Input: dimensioned drawing with shaded views. Units: mm. Origin: part minimum x, y, z. Coordinates: 2 decimals unless noted, no trailing zeros. Order: outer loops, then holes, each group sorted by start corner. A loop starts at its lowest first (then second) coordinate and runs counter-clockwise, first axis right, second up. Notation, with made-up numbers: (88.5, 66) -> (95.5, 66) arc R25 cw to (95.5, 80) -> close; hole circle Ø11 at (70, -20). An arc over 180 degrees is marked (long way). Write item = value, one per line. Start each with the question number.
Item 1: Section query A-A (x = 38). Output: boundary loops of the cut face in (y, z), then the cut area to 3 significant figures.
Item 2: Section query D-D (x = 51). Output: boundary loops of the cut face in (y, z), then the cut area to 3 significant figures.
Item 3: Section query B-B (z = 38). Output: boundary loops of the cut face in (x, y).
Item 4: Contact query for flat-ended pins moving along their axis: pin 1 (5 mm diameter, centred on y = 7.5, z = 50, fed in from +X); pin 2 (3 mm diameter, centred on y = 5.5, z = 41.5, fed in from +X); pin 3 (1.5 mm diameter, centred on x = 61, y = 7, fed in from +Z) (1 decimal). Output: stop coordinate, or through.
Item 5: Section query C-C (z = 29). Output: boundary loops of the cut face in (x, y).
Item 6: Ray query, line 1 along X through (y, z) = (4.5, 38); line 2 along Z through (x, y) = (21.5, 8); line 3 along Z through (x, y) = (21, 1.75) (1 decimal). Return the intervals inside material, ascending. Write a range as [from, to].
Item 7: Mould query, pull axis Z, two halves, no side actions, for the marked faces 1, 2 and 3. Classes: released by +Z, released by -Z, zero draft, split by the parting line, or undercut.
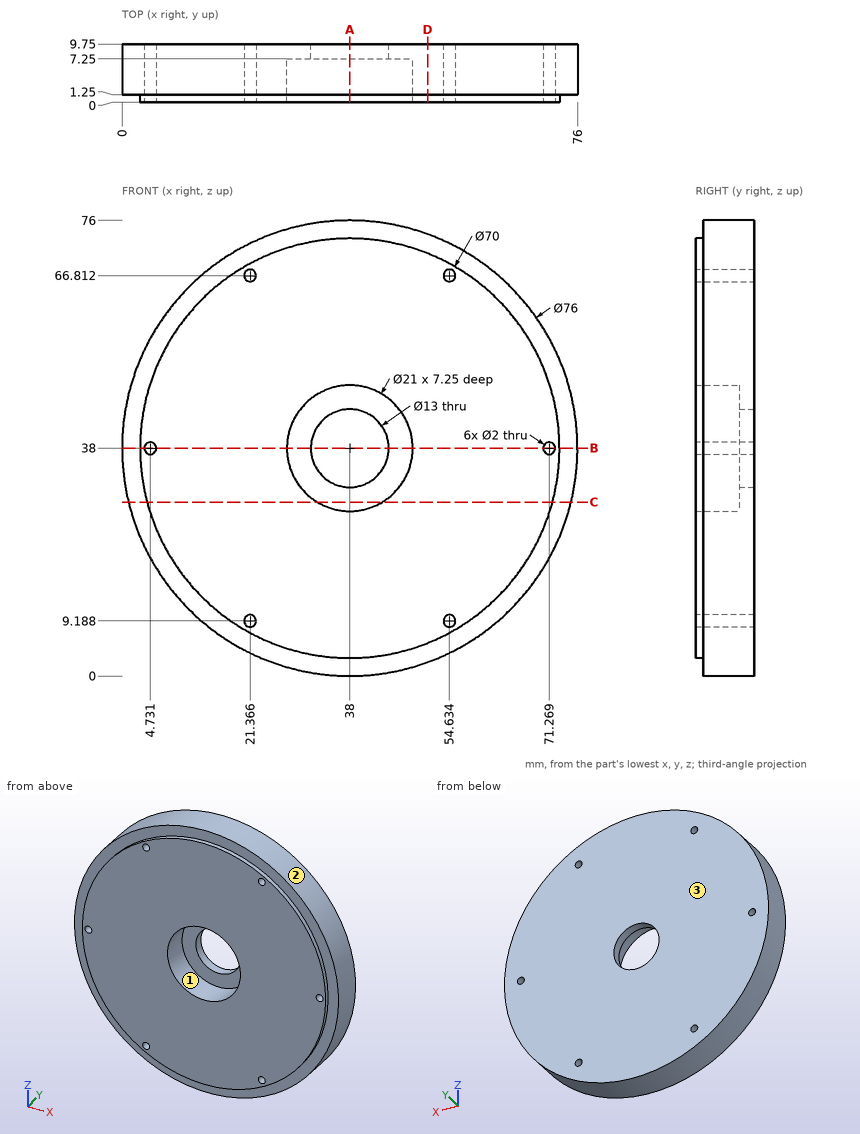
Computed:
q1.outline = (0, 3) -> (1.25, 3) -> (1.25, 0) -> (9.75, 0) -> (9.75, 31.5) -> (7.25, 31.5) -> (7.25, 27.5) -> (0, 27.5) -> close; (0, 48.5) -> (7.25, 48.5) -> (7.25, 44.5) -> (9.75, 44.5) -> (9.75, 76) -> (1.25, 76) -> (1.25, 73) -> (0, 73) -> close
q1.area = 549 mm^2
q2.outline = (0, 5.5) -> (1.25, 5.5) -> (1.25, 2.29) -> (9.75, 2.29) -> (9.75, 73.71) -> (1.25, 73.71) -> (1.25, 70.5) -> (0, 70.5) -> close
q2.area = 688 mm^2
q3.outline = (0, 1.25) -> (3, 1.25) -> (3, 0) -> (3.73, 0) -> (3.73, 9.75) -> (0, 9.75) -> close; (5.73, 0) -> (27.5, 0) -> (27.5, 7.25) -> (31.5, 7.25) -> (31.5, 9.75) -> (5.73, 9.75) -> close; (44.5, 7.25) -> (48.5, 7.25) -> (48.5, 0) -> (70.27, 0) -> (70.27, 9.75) -> (44.5, 9.75) -> close; (72.27, 0) -> (73, 0) -> (73, 1.25) -> (76, 1.25) -> (76, 9.75) -> (72.27, 9.75) -> close
q4.pin_1 = 74.79
q4.pin_2 = 75.95
q4.pin_3 = 68.8
q5.outline = (1.08, 1.25) -> (4.18, 1.25) -> (4.18, 0) -> (32.59, 0) -> (32.59, 7.25) -> (43.41, 7.25) -> (43.41, 0) -> (71.82, 0) -> (71.82, 1.25) -> (74.92, 1.25) -> (74.92, 9.75) -> (1.08, 9.75) -> close
q6.line_1 = [0, 3.73], [5.73, 27.5], [48.5, 70.27], [72.27, 76]
q6.line_2 = [3.77, 8.2], [10.18, 65.82], [67.8, 72.23]
q6.line_3 = [4, 8.3], [10.1, 65.9], [67.7, 72]
q7.face_1 = undercut
q7.face_2 = split by the parting line
q7.face_3 = zero draft
